Read the model definition and answer for the solid it produces. Units are mm, in the model's axes. A direction names the side the tool comes from. Coordinates: 2 decimals unless noted, no trailing zeros. Loops run counter-clockwise (first coordinate to the right, second up) from the corner with the lowest first, then second, coordinate; pieces in that order, holes last. Notation, with made-up numbers: (20, -35.5) -> (73, -35.5) arc R18 ccw to (73, -20.5) -> close; hole circle Ø5 at (89, 74). An arc over 180 degrees is marked (long way). Answer in a Markdown table with one row per item.
```python
from build123d import *

# Parameters (mm, degrees)
SKETCH_W        = 110
SKETCH_H        = 50
PAD_DEPTH       = 3
SKETCH001_W     = 8
SKETCH001_H     = 50
PAD001_DEPTH    = 5
SKETCH002_R     = 2
POCKET_DEPTH    = 10
SKETCH003_R     = 2
POCKET001_DEPTH = 10
SKETCH004_R     = 2
POCKET002_DEPTH = 10
SKETCH005_R     = 2
POCKET003_DEPTH = 10


with BuildPart() as part:
    # Sketch → Pad (new body)
    with BuildSketch(Plane.XY):
        Rectangle(SKETCH_W, SKETCH_H)
    extrude(amount=PAD_DEPTH)

    # Sketch001 (on Face6 of Pad) → Pad001 (join)
    with BuildSketch(Plane.XY.offset(3)):
        with Locations((51, 0)):
            Rectangle(SKETCH001_W, SKETCH001_H)
        with Locations((-51, 0)):
            Rectangle(SKETCH001_W, SKETCH001_H)
    extrude(amount=PAD001_DEPTH)

    # Sketch002 (on Face5 of Pad001) → Pocket (cut)
    with BuildSketch(Plane(origin=(0, 25, 0), x_dir=(-1, 0, 0), z_dir=(0, 1, 0))):
        with Locations((51, 4)):
            Circle(SKETCH002_R)
        with Locations((-51, 4)):
            Circle(SKETCH002_R)
    extrude(amount=-POCKET_DEPTH, mode=Mode.SUBTRACT)

    # Sketch003 (on Face20 of Pocket) → Pocket001 (cut)
    with BuildSketch(Plane.XZ.offset(25)):
        with Locations((-51, 4)):
            Circle(SKETCH003_R)
        with Locations((51, 4)):
            Circle(SKETCH003_R)
    extrude(amount=-POCKET001_DEPTH, mode=Mode.SUBTRACT)

    # Sketch004 (on Face17 of Pocket001) → Pocket002 (cut)
    with BuildSketch(Plane(origin=(-55, 0, 0), x_dir=(0, -1, 0), z_dir=(-1, 0, 0))):
        with Locations((0, 4)):
            Circle(SKETCH004_R)
    extrude(amount=-POCKET002_DEPTH, mode=Mode.SUBTRACT)

    # Sketch005 (on Face11 of Pocket002) → Pocket003 (cut)
    with BuildSketch(Plane.YZ.offset(55)):
        with Locations((0, 4)):
            Circle(SKETCH005_R)
    extrude(amount=-POCKET003_DEPTH, mode=Mode.SUBTRACT)


solid = part.part
```
1. A cutting plane is placed at A-A on z = 4. Count the separate pieces of the cut face and the enclosed holes in it, and give its area (3 significant figures).
A:
| item | result |
|---|---|
| separate pieces | 4 |
| enclosed holes | 0 |
| area | 576 mm2 |
2. A cutting plane is placed at B-B on y = 0. Give the vertices of the cut face in (x, z).
A:
| item | result |
|---|---|
| outline | (-55, 0) -> (55, 0) -> (55, 2) -> (45, 2) -> (45, 3) -> (-45, 3) -> (-45, 2) -> (-55, 2) -> close; (-55, 6) -> (-47, 6) -> (-47, 8) -> (-55, 8) -> close; (47, 6) -> (55, 6) -> (55, 8) -> (47, 8) -> close |
3. A cutting plane is placed at D-D on x = 51. Give the vertices of the cut face in (y, z), and give its area (3 significant figures).
A:
| item | result |
|---|---|
| outline | (-25, 0) -> (25, 0) -> (25, 2) -> (15, 2) -> (15, 6) -> (25, 6) -> (25, 8) -> (-25, 8) -> (-25, 6) -> (-15, 6) -> (-15, 2) -> (-25, 2) -> close; hole circle Ø4 at (0, 4) |
| area | 307 mm2 |
4. The mould has two halves that part along Y. Classify faces 6 (the cylindrical face through (51, 0, 2)), 7 (the flat face through (-1, 25, 2)), 8 (the cylindrical face through (-51, 0, 2)), 9 (the flat face through (-1, 0, 3)): pulls with the +Y half, pulls with the -Y half, needs draft (parallel to the pull), parting line crosses it, or undercut.
A:
| item | result |
|---|---|
| face 6 | undercut |
| face 7 | pulls with the +Y half |
| face 8 | undercut |
| face 9 | needs draft |
5. A cutting plane is placed at C-C on y = -16. Give the vertices of the cut face in (x, z), and give its area (3 significant figures).
A:
| item | result |
|---|---|
| outline | (-55, 0) -> (55, 0) -> (55, 8) -> (47, 8) -> (47, 3) -> (-47, 3) -> (-47, 8) -> (-55, 8) -> close; hole circle Ø4 at (-51, 4); hole circle Ø4 at (51, 4) |
| area | 385 mm2 |
6. Find the intervals of material crossed by probe 1 along X at (y, z) = (-21.5, 4.25); probe 2 along Z at (x, y) = (48, 0); probe 3 along X at (y, z) = (-18.5, 3.5), in increasing order.
A:
| item | result |
|---|---|
| probe 1 | x = -55 to -52.98, -49.02 to -47, 47 to 49.02, 52.98 to 55 |
| probe 2 | z = 0 to 2, 6 to 8 |
| probe 3 | x = -55 to -52.94, -49.06 to -47, 47 to 49.06, 52.94 to 55 |
7. A tool of negligible diameter and unlimited length cuts with its end or side. For faces 1 (the cylindrical face through (-49.153, -20.07, 3.234)), 2 (the flat face through (47, 0, 7)), 3 (the flat face through (51, 0, 8)), 4 (the flat face through (55, 0, 7)), 5 (the cylindrical face through (49.153, 20.07, 3.234)), from which of +Z, -Z, +X, -X, +Y, -Y can it reach the whole face along a straight path? Write none if from no direction.
A:
| item | result |
|---|---|
| face 1 | -Y |
| face 2 | +Z, +Y, -Y |
| face 3 | +Z, +X, -X, +Y, -Y |
| face 4 | +Z, -Z, +X, +Y, -Y |
| face 5 | +Y |
8. Given pin 1 Ø4 at (x, y) = (32, -2.5) entering from +Z; pin 2 Ø3.5 at (y, z) = (0, 4) entering from -X; pin 3 Ø1.2 at (x, z) = (-50.5, 4) entering from -Y; pin 4 Ø1.5 at (x, z) = (9.5, 5.5) entering from -Y, each flat-ended and moving along its own axis, determine where each tip first touches the part or whether it passes through.
A:
| item | result |
|---|---|
| pin 1 | stops at z = 3 |
| pin 2 | stops at x = -45 |
| pin 3 | stops at y = -15 |
| pin 4 | passes through |
